from build123d import *

# Parameters (mm, degrees)
SKETCH1_W           = 24.634
SKETCH1_H           = 13
BOSS_EXTRUDE1_DEPTH = 10
SKETCH4_W           = 82.5
SKETCH4_H           = 13
BOSS_EXTRUDE4_DEPTH = 15
SKETCH5_W           = 28
SKETCH5_H           = 3.5
BOSS_EXTRUDE5_DEPTH = 15
CUT_EXTRUDE1_DEPTH  = 88.769584709
SKETCH7_W           = 32.5
SKETCH7_H           = 5
CUT_EXTRUDE2_DEPTH  = 2
SKETCH11_R          = 2.68
CUT_EXTRUDE3_DEPTH  = 88.769584709
FILLET1_R           = 10
FILLET2_R           = 5
BOSS_EXTRUDE6_DEPTH = 3.5


with BuildPart() as part:
    # Sketch1 → Boss-Extrude1 (new body)
    with BuildSketch(Plane.XY):
        with Locations((12.317, 6.5)):
            Rectangle(SKETCH1_W, SKETCH1_H)
    extrude(amount=BOSS_EXTRUDE1_DEPTH)

    # Sketch4 → Boss-Extrude4 (add)
    with BuildSketch(Plane.XY.offset(10)):
        with Locations((41.25, 6.5)):
            Rectangle(SKETCH4_W, SKETCH4_H)
    extrude(amount=BOSS_EXTRUDE4_DEPTH)

    # Sketch5 → Boss-Extrude5 (add)
    with BuildSketch(Plane.XY.offset(25)):
        with Locations((68.5, -1.75)):
            Rectangle(SKETCH5_W, SKETCH5_H)
        with Locations((68.5, 14.75)):
            Rectangle(SKETCH5_W, SKETCH5_H)
    extrude(amount=-BOSS_EXTRUDE5_DEPTH)

    # Sketch6 → Cut-Extrude1 (cut, through all)
    with BuildSketch(Plane.XY.offset(25)):
        with BuildLine():
            Line((63.16, 9.16), (69.84, 9.16))
            ThreePointArc((69.84, 9.16), (72.5, 6.5), (69.84, 3.84))
            Line((69.84, 3.84), (63.16, 3.84))
            ThreePointArc((63.16, 3.84), (60.5, 6.5), (63.16, 9.16))
        make_face()
    extrude(amount=-CUT_EXTRUDE1_DEPTH, mode=Mode.SUBTRACT)

    # Sketch7 → Cut-Extrude2 (cut)
    with BuildSketch(Plane.XY.offset(25)):
        with Locations((66.25, 6.5)):
            Rectangle(SKETCH7_W, SKETCH7_H)
    extrude(amount=-CUT_EXTRUDE2_DEPTH, mode=Mode.SUBTRACT)

    # Sketch11 → Cut-Extrude3 (cut, through all)
    with BuildSketch(Plane(origin=(0, 0, 0), x_dir=(-1, 0, 0), z_dir=(0, 0, -1))):
        with Locations((-5.067, 6.5)):
            Circle(SKETCH11_R)
        with Locations((-19.567, 6.5)):
            Circle(SKETCH11_R)
    extrude(amount=-CUT_EXTRUDE3_DEPTH, mode=Mode.SUBTRACT)

    # Fillet1
    # the kernel refuses this fillet: 10 mm, written as the material it adds along each edge
    with BuildSketch(Plane(origin=(54.5, 13, 25), x_dir=(-1, 0, 0), z_dir=(0, 0, -1))) as fillet1_piece_1:
        with BuildLine():
            CenterArc((7.599342077, 10), FILLET1_R, 220.541601874, 49.458398126)
            Line((0, 3.5), (-0.151986842, 3.37))
            ThreePointArc((-0.151986842, 3.37), (-0.2, 1.75), (-0.2, 0))
            Line((-0.2, 0), (0, -0.2))
            Line((0, -0.2), (7.599342077, -0.2))
            Line((7.599342077, -0.2), (7.599342077, 0))
        make_face()
    extrude(amount=15)
    with BuildSketch(Plane(origin=(54.5, 0, 25), x_dir=(-1, 0, 0), z_dir=(0, 0, -1))) as fillet1_piece_2:
        with BuildLine():
            CenterArc((7.599342077, -10), FILLET1_R, 90, 49.458398126)
            Line((0, -3.5), (-0.151986842, -3.37))
            ThreePointArc((-0.151986842, -3.37), (-0.2, -1.75), (-0.2, 0))
            Line((-0.2, 0), (0, 0.2))
            Line((0, 0.2), (7.599342077, 0.2))
            Line((7.599342077, 0.2), (7.599342077, 0))
        make_face()
    extrude(amount=15)

    # Fillet2
    fillet2_edges = [part.edges().sort_by_distance(p)[0] for p in [
        (24.634, 6.5, 10),
    ]]
    fillet(fillet2_edges, radius=FILLET2_R)

    # Sketch12 → Boss-Extrude6 (add)
    with BuildSketch(Plane(origin=(82.5, 0, 0), x_dir=(0, 0, -1), z_dir=(1, 0, 0))):
        Polygon((-25, 16.5), (-25, 9), (-23, 9), (-23, 4), (-25, 4), (-25, -3.5), (-10, -3.5), (-10, 16.5), align=None)
    extrude(amount=BOSS_EXTRUDE6_DEPTH)


solid = part.part
Model file for the job. Use its own axes, mm. A direction names the side the tool comes from. Give positions to 0.01 mm unless a question says otherwise; leave off trailing zeros. Loops run counter-clockwise (first coordinate to the right, second up) from the corner with the lowest first, then second, coordinate; pieces in that order, holes last.
Item 1: Slice it at D-D (z = 8.25). Write the cut outline in (x, y).
Check values:
outline: (0, 0) - (25.83, 0) - (25.83, 13) - (0, 13) - close; hole circle Ø5.36 at (5.07, 6.5); hole circle Ø5.36 at (19.57, 6.5)
Item 2: Slice it at A-A (z = 17.25). Write the cut outline in (x, y).
Check values:
outline: (0, 0) - (46.9, 0) arc R10 cw to (54.5, -3.5) - (86, -3.5) - (86, 16.5) - (54.5, 16.5) arc R10 cw to (46.9, 13) - (0, 13) - close; hole circle Ø5.36 at (5.07, 6.5); hole circle Ø5.36 at (19.57, 6.5); hole (63.16, 3.84) - (69.84, 3.84) arc R2.66 ccw to (69.84, 9.16) - (63.16, 9.16) arc R2.66 ccw to start
Item 3: Which spindle directions (+Z, -Z, +X, -X, +Y, -Y) get a long thin tool onto all of the face, cutting with end or side? Do faces 5 (the face through (24.634, 6, 2)), 6 (the face through (18, 0, 15)), 7 (the face through (78, 9, 24)), 8 (the face through (17.01, 7.3, 12.32)), 9 (the face through (70, 16.5, 17)). Say none if no direction does.
Check values:
face 5: -Z, +X, +Y, -Y
face 6: +Z, -Z, -X, -Y
face 7: +Z, +X
face 8: +Z, -Z
face 9: +Z, -Z, +X, -X, +Y
Item 4: Drop flat-ended pins along their axis: P1, Ø12.5, axis at x = 31, z = 9.5, coming from the -Y side; P2, Ø5.5, axis at y = 5, z = 2.5, coming from the +X side; P3, Ø5, axis at x = 5.067, y = 6.5, coming from the -Z side; P4, Ø1.6, axis at y = 5.5, z = 24, coming from the +X side. Give the stop position or say it passes through.
Check values:
P1: stops at y = 0
P2: stops at x = 24.64
P3: passes through
P4: stops at x = 50
Item 5: Slice it at B-B (y = 6.5). Write the cut outline in (x, z).
Check values:
outline: (0, 0) - (2.39, 0) - (2.39, 25) - (0, 25) - close; (7.75, 0) - (16.89, 0) - (16.89, 25) - (7.75, 25) - close; (22.25, 0) - (24.63, 0) - (24.63, 5) arc R5 cw to (29.63, 10) - (60.5, 10) - (60.5, 23) - (50, 23) - (50, 25) - (22.25, 25) - close; (72.5, 10) - (86, 10) - (86, 23) - (72.5, 23) - close
Item 6: Mould opens along X. For faces 1 (the face through (72.5, 6.6, 17.6)), 2 (the face through (50, 6, 24)), 3 (the face through (67, 3.84, 18)), 4 (the face through (56, 4, 24)) say: +X half, -X half, draft (parallel to the pull), parting line (faces both ways), or undercut.
Check values:
face 1: undercut
face 2: +X half
face 3: undercut
face 4: draft
Item 7: Slice it at C-C (y = 12.25). Write the cut outline in (x, z), plus the area to 3 significant figures.
Check values:
outline: (0, 0) - (24.63, 0) - (24.63, 5) arc R5 cw to (29.63, 10) - (86, 10) - (86, 25) - (0, 25) - close
area: 1,540 mm2
Item 8: Drill centre lines: line 1 along X through (y, z) = (4.75, 11.75); line 2 along Y through (x, z) = (69.5, 21.75); line 3 along X through (y, z) = (8.5, 4). Where is each one in solid material? Low to high.
Check values:
line 1: x = 0 to 3.04, 7.1 to 17.54, 21.6 to 61.16, 71.84 to 86
line 2: y = -3.5 to 3.84, 9.16 to 16.5
line 3: x = 0 to 3.28, 6.85 to 17.78, 21.35 to 24.63
